```python
from build123d import *

# Parameters (mm, degrees)
SKETCH1_R           = 4.25
BOSS_EXTRUDE1_DEPTH = 2


with BuildPart() as part:
    # Sketch1 → Boss-Extrude1 (new body)
    with BuildSketch(Plane(origin=(0, 0, 0), x_dir=(1, 0, 0), z_dir=(0, 1, 0))):
        with BuildLine():
            Line((-39.5, 7), (-17, 7))
            ThreePointArc((-17, 7), (-9.928932188, 9.928932188), (-7, 17))
            Line((-7, 17), (-7, 39.5))
            ThreePointArc((-7, 39.5), (0, 46.5), (7, 39.5))
            Line((7, 39.5), (7, 17))
            ThreePointArc((7, 17), (9.928932188, 9.928932188), (17, 7))
            Line((17, 7), (39.5, 7))
            ThreePointArc((39.5, 7), (46.5, 0), (39.5, -7))
            Line((39.5, -7), (17, -7))
            ThreePointArc((17, -7), (9.928932188, -9.928932188), (7, -17))
            Line((7, -17), (7, -39.5))
            ThreePointArc((7, -39.5), (0, -46.5), (-7, -39.5))
            Line((-7, -39.5), (-7, -17))
            ThreePointArc((-7, -17), (-9.928932188, -9.928932188), (-17, -7))
            Line((-17, -7), (-39.5, -7))
            ThreePointArc((-39.5, -7), (-46.5, 0), (-39.5, 7))
        make_face()
        with Locations(Location((0, 39.5, 0), (0, 0, 270))):
            Circle(SKETCH1_R, mode=Mode.SUBTRACT)
        with Locations(Location((39.5, 0, 0), (0, 0, 270))):
            Circle(SKETCH1_R, mode=Mode.SUBTRACT)
        with Locations(Location((0, -39.5, 0), (0, 0, 270))):
            Circle(SKETCH1_R, mode=Mode.SUBTRACT)
        with Locations(Location((-39.5, 0, 0), (0, 0, 270))):
            Circle(SKETCH1_R, mode=Mode.SUBTRACT)
    extrude(amount=BOSS_EXTRUDE1_DEPTH)


solid = part.part
```
Can you work these out from the model? Positions are in its coordinate system, mm. A direction names the side the tool comes from. Coordinates: 2 decimals unless noted, no trailing zeros. Order: outer loops, then holes, each group sorted by start corner. A loop starts at its lowest first (then second) coordinate and runs counter-clockwise, first axis right, second up.
1. If we section it at A-A (z = 0): Please give me the cut outline in (x, y).
2. If we section it at D-D (z = -23): Please give me the cut outline in (x, y), then the cut area to 3 significant figures.
3. If we section it at B-B (y = 1.2): Please give me the cut outline in (x, z).
4. For faces 1 (the face through (7, 1, 28)), 2 (the face through (-7, 1, 28)), 3 (the face through (28, 1, -7)), which set-ups out of +Z, -Z, +X, -X, +Y, -Y let a thin tool reach every point of the face, with its end or its side?
5. I need wall thicknesses on line 1 (X direction, y = 0.45, z = 0); line 2 (X direction, y = 0.3, z = 2.5); line 3 (Z direction, x = -25, y = 1.85). Which ranges of each line are inside material? Lowest first, please.
6. Thinking about a two-plate mould opening in X: for faces 4 (the face through (7, 1, -28)), 5 (the face through (-35.286, 0.986, -0.553)), 6 (the face through (-28, 1, 7)), which applies, +X half, -X half, draft (parallel to the pull), parting line (faces both ways), or undercut?
7. If we section it at C-C (x = -19): Please give me the cut outline in (y, z).
8. I'm going to push flat-ended pins straight in: pin 1 (1 mm diameter, centred on x = -4.5, y = 0.5, fed in from -Z); pin 2 (1 mm diameter, centred on y = 0.5, z = 14.5, fed in from +X); pin 3 (1 mm diameter, centred on x = -23.5, y = 0.5, fed in from +Z). Where does each tip first touch, or does it pass through?
Entries:
1. outline: (-46.5, 0) - (-43.75, 0) - (-43.75, 2) - (-46.5, 2) - close; (-35.25, 0) - (35.25, 0) - (35.25, 2) - (-35.25, 2) - close; (43.75, 0) - (46.5, 0) - (46.5, 2) - (43.75, 2) - close
2. outline: (-7, 0) - (7, 0) - (7, 2) - (-7, 2) - close
2. area: 28.0 mm2
3. outline: (-39.5, -7) - (-17, -7) arc R10 cw to (-7, -17) - (-7, -39.5) arc R7 ccw to (7, -39.5) - (7, -17) arc R10 cw to (17, -7) - (39.5, -7) arc R7 ccw to (39.5, 7) - (17, 7) arc R10 cw to (7, 17) - (7, 39.5) arc R7 ccw to (-7, 39.5) - (-7, 17) arc R10 cw to (-17, 7) - (-39.5, 7) arc R7 ccw to start; hole circle Ø8.5 at (-39.5, 0); hole circle Ø8.5 at (0, -39.5); hole circle Ø8.5 at (0, 39.5); hole circle Ø8.5 at (39.5, 0)
4. face 1: +Z, +X, +Y, -Y
4. face 2: +Z, -X, +Y, -Y
4. face 3: -Z, +X, +Y, -Y
5. line 1: x = -46.5 to -43.75, -35.25 to 35.25, 43.75 to 46.5
5. line 2: x = -46.04 to -42.94, -36.06 to 36.06, 42.94 to 46.04
5. line 3: z = -7 to 7
6. face 4: +X half
6. face 5: undercut
6. face 6: draft
7. outline: (0, -7) - (2, -7) - (2, 7) - (0, 7) - close
8. pin 1: stops at z = -45.24
8. pin 2: stops at x = 7.46
8. pin 3: stops at z = 7
